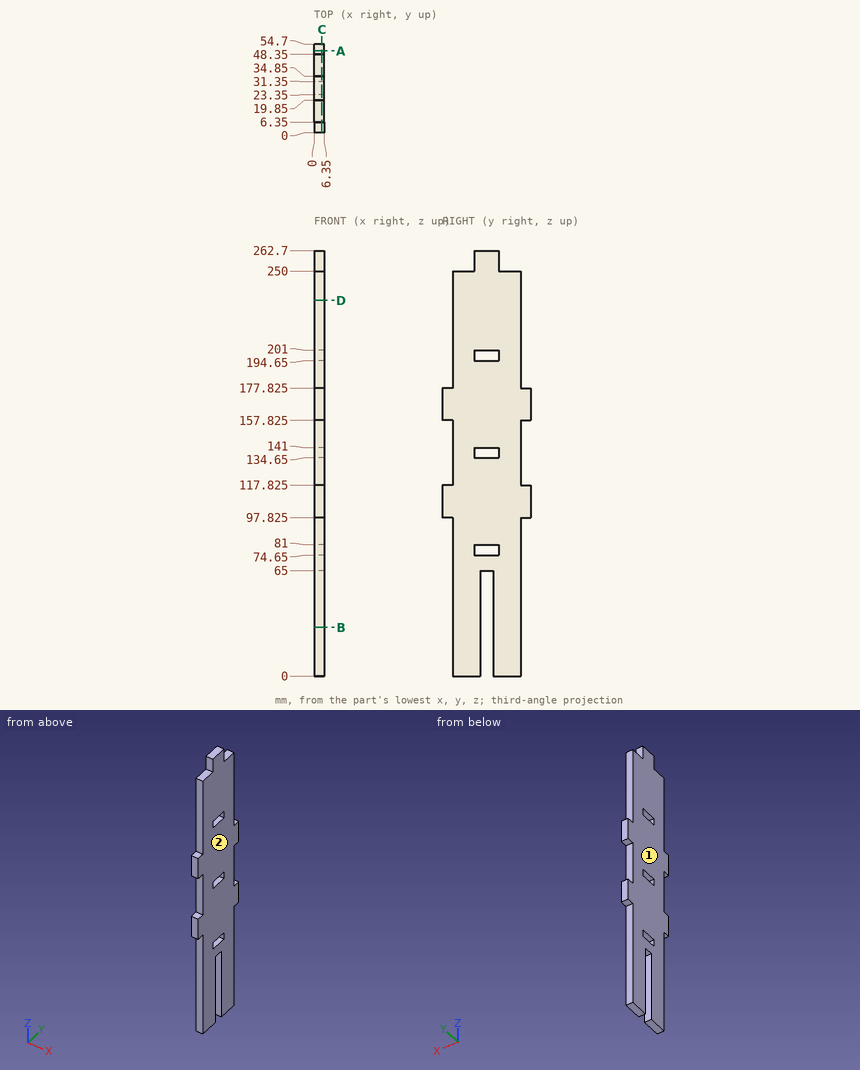
The figure shows three views and two pictorial views of one solid part (mm, origin at its lowest corner). Answer the questions. Round coordinates to 2 decimals unless told otherwise and drop trailing zeros. Loops run counter-clockwise (first coordinate to the right, second up) from the corner with the lowest first, then second, coordinate; pieces in that order, holes last. Notation, with made-up numbers: M -3.5,50.25 L 26.5,50.25 A18 ccw 26.5,67.25 Z; hole C -9.75,-36.5 d6. An arc over 180 degrees is marked long. Return JSON: item names as keys, results as strings.
Q1. Find section C-C, the plane x = 4.75. State how many separate pieces and enclosed holes the cut face has, plus the area to 3 significant figures.
Results list:
{"separate pieces": "1", "enclosed holes": "3", "area": "10,400 mm2"}
Q2. Each of these flat-tipped pins is pushed along its axis until it touches: pin 1 Ø1.9 at (x, y) = (4, 50.5) entering from +Z (3 decimals); pin 2 Ø3 at (x, z) = (2, 55) entering from -Y; pin 3 Ø3 at (x, y) = (2, 41) entering from +Z. Where does it stop, or does it pass through?
Results list:
{"pin 1": "stops at z = 177.825", "pin 2": "stops at y = 6.35", "pin 3": "stops at z = 250"}
Q3. Find the intervals of material crossed by line 1 along Z through (x, y) = (5.25, 29); line 2 along Y through (x, z) = (5.5, 80); line 3 along Y through (x, z) = (1, 29.5), in increasing order. Write a range as from..to.
Results list:
{"line 1": "z = 65..74.65, 81..134.65, 141..194.65, 201..262.7", "line 2": "y = 6.35..19.85, 34.85..48.35", "line 3": "y = 6.35..23.35, 31.35..48.35"}
Q4. Find section D-D, the plane z = 232. Determine the outline of the cut face in (x, y).
Results list:
{"outline": "M 0,6.35 L 6.35,6.35 L 6.35,48.35 L 0,48.35 Z"}
Q5. Find section A-A, the plane y = 50.5. Determine the outline of the cut face in (x, z) (3 decimals), plus the area to 3 significant figures.
Results list:
{"outline": "M 0,97.825 L 6.35,97.825 L 6.35,117.825 L 0,117.825 Z; M 0,157.825 L 6.35,157.825 L 6.35,177.825 L 0,177.825 Z", "area": "254 mm2"}
Q6. The mould has two halves that part along X. Classify the marked faces 1 and 2: released by +X, released by -X, zero draft, split by the parting line, or undercut.
Results list:
{"face 1": "released by -X", "face 2": "released by +X"}
Q7. Find section B-B, the plane z = 30. Determine the outline of the cut face in (x, y), plus the area to 3 significant figures.
Results list:
{"outline": "M 0,6.35 L 6.35,6.35 L 6.35,23.35 L 0,23.35 Z; M 0,31.35 L 6.35,31.35 L 6.35,48.35 L 0,48.35 Z", "area": "216 mm2"}
